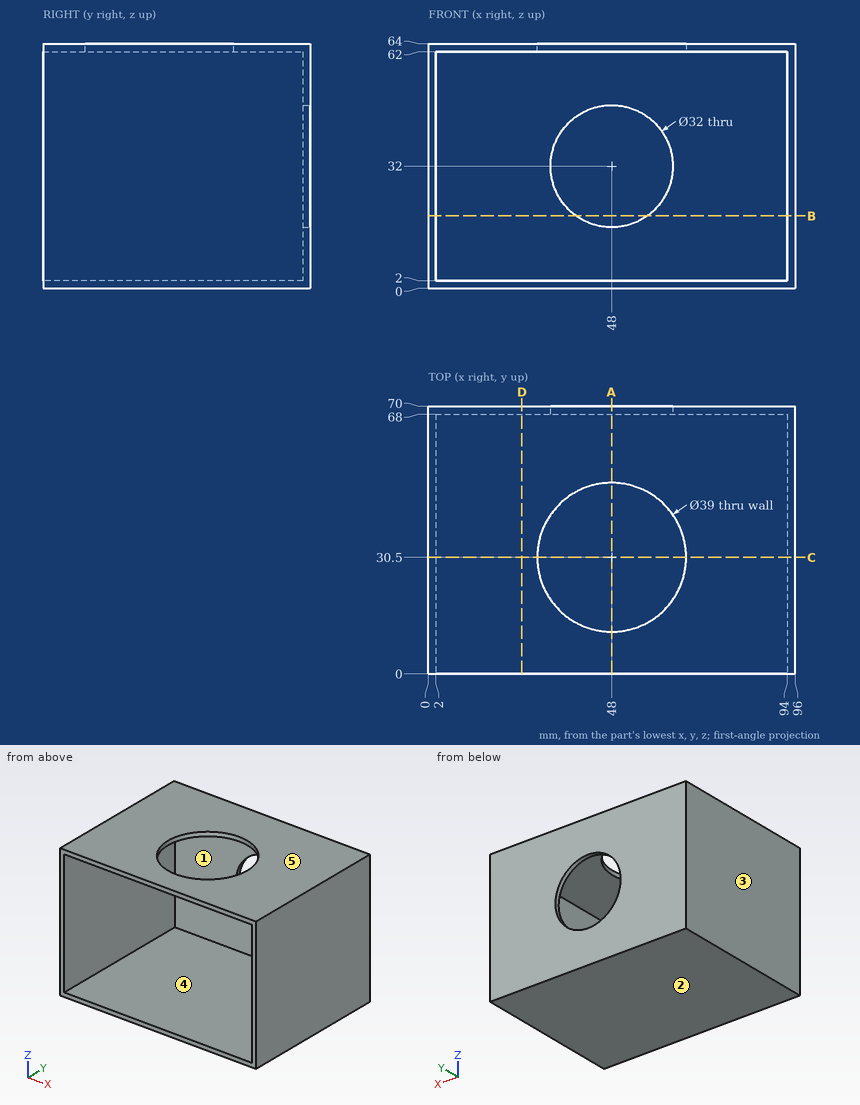
Geometry check sheet. Reference: drawing and pictorial views, mm from the part's lowest x, y, z. A direction names the side the tool comes from. Coordinates: 2 decimals unless noted, no trailing zeros. Order: outer loops, then holes, each group sorted by start corner. A loop starts at its lowest first (then second) coordinate and runs counter-clockwise, first axis right, second up. Notation, with made-up numbers: (73.25, 55) - (123.25, 55) arc R18 ccw to (123.25, 79) - close; hole circle Ø10 at (86.25, 18). An arc over 180 degrees is marked (long way). One line per item, written item: value.
(1) Access from +Z, -Z, +X, -X, +Y, -Y to the whole of each face (thin tool, end or side, straight path). Record for the marked faces 4 and 5.
Data:
face 4: -Y
face 5: +Z, +X, -X, +Y, -Y
(2) Sectioned sample at A-A (x = 48). Enter the section's corners in (y, z), and give its area (3 significant figures).
Data:
outline: (0, 0) - (70, 0) - (70, 16) - (68, 16) - (68, 2) - (0, 2) - close; (0, 62) - (11, 62) - (11, 64) - (0, 64) - close; (50, 62) - (68, 62) - (68, 48) - (70, 48) - (70, 64) - (50, 64) - close
area: 258 mm^2
(3) Thickness scan on probe 1 along Y at (x, z) = (48, 63); probe 2 along Z at (x, y) = (90, 6.5); probe 3 along X at (y, z) = (20.5, 37). Record the ranges inside material, lowest first. Write a range as from..to.
Data:
probe 1: y = 0..11, 50..70
probe 2: z = 0..2, 62..64
probe 3: x = 0..2, 94..96
(4) Sectioned sample at D-D (x = 24.5). Enter the section's corners in (y, z).
Data:
outline: (0, 0) - (70, 0) - (70, 64) - (0, 64) - (0, 62) - (68, 62) - (68, 2) - (0, 2) - close
(5) Sectioned sample at C-C (y = 30.5). Enter the section's corners in (x, z), and give its area (3 significant figures).
Data:
outline: (0, 0) - (96, 0) - (96, 64) - (67.5, 64) - (67.5, 62) - (94, 62) - (94, 2) - (2, 2) - (2, 62) - (28.5, 62) - (28.5, 64) - (0, 64) - close
area: 546 mm^2
(6) Sectioned sample at B-B (z = 19). Enter the section's corners in (x, y), and give its area (3 significant figures).
Data:
outline: (0, 0) - (2, 0) - (2, 68) - (38.67, 68) - (38.67, 70) - (0, 70) - close; (57.33, 68) - (94, 68) - (94, 0) - (96, 0) - (96, 70) - (57.33, 70) - close
area: 427 mm^2
(7) Depth check by flat-ended pin: pin 1 Ø3 at (x, z) = (12.5, 16.5) entering from -Y; pin 2 Ø3 at (x, y) = (43, 25.5) entering from +Z. Enter the tip coordinate at first touch or a pass-through.
Data:
pin 1: stops at y = 68
pin 2: stops at z = 2
(8) Release check for a two-part mould opening along Z. For the marked faces 1, 2 and 3 record: +Z half, -Z half, draft (parallel to the pull), parting line (faces both ways), or undercut.
Data:
face 1: undercut
face 2: -Z half
face 3: draft
